```python
from build123d import *

# Parameters (mm, degrees)
F1_W     = 101.6
F1_H     = 101.6
F2_DEPTH = 50.8
F3_W     = 26.3578668237
F3_H     = 22.6122755557
F4_DEPTH = 50.8
F5_R     = 17.6293811016
F6_DEPTH = 50.8
F8_DEPTH = 50.8


# Not quite as in the source:
# - a variable given as a bare number and used for a length is read in inches; the dataset says mm whatever the document's units were


with BuildPart() as f2:
    # F1 (on Front) → F2 (new body, symmetric)
    with BuildSketch(Plane.XZ):
        Rectangle(F1_W, F1_H)
    extrude(amount=F2_DEPTH, both=True)

    # F3 (on face) → F4 (cut)
    with BuildSketch(Plane.XY.offset(50.8)):
        Rectangle(F3_W, F3_H)
    extrude(amount=-F4_DEPTH, mode=Mode.SUBTRACT)

    # F5 (on face) → F6 (cut)
    with BuildSketch(Plane(origin=(0, 0, -50.8), x_dir=(1, 0, 0), z_dir=(0, 0, -1))):
        with Locations((0, 1.7344856169)):
            Circle(F5_R)
    extrude(amount=-F6_DEPTH, mode=Mode.SUBTRACT)

    # F7 (on face) → F8 (cut)
    with BuildSketch(Plane(origin=(-50.8, 0, 0), x_dir=(0, -1, 0), z_dir=(-1, 0, 0))):
        Polygon((26.357864961, -15.2177204305), (26.357864961, 15.2177204305), (0, 30.435440861), (-26.357864961, 15.2177204305), (-26.357864961, -15.2177204305), (0, -30.435440861), align=None)
    extrude(amount=-F8_DEPTH, mode=Mode.SUBTRACT)


solid = f2.part
```
CAD build for the part. Positions are in the model's coordinates, mm. A direction names the side the tool comes from. Coordinates: 2 decimals unless noted, no trailing zeros. Write each loop counter-clockwise with the first axis right and the second up, starting at its lowest first coordinate (ties: lowest second). Pieces come first, ordered by that corner, then holes. Notation, with made-up numbers: (58, 74.25) -> (68, 74.25) arc R20 cw to (68, 87.25) -> close; hole circle Ø1 at (52, 20.5). An arc over 180 degrees is marked (long way). Use CSV: the item, a comma, the result in double quotes. Start each with the question number.
Item 1: Band-saw the part on B-B, the plane y = -6. Write the cut outline in (x, z), plus the area to 3 significant figures.
Item 2: Drop flat-ended pins along their axis: P1, Ø1.4, axis at x = 7.5, y = 13, coming from the -Z side; P2, Ø18, axis at y = -4, z = 15.5, coming from the -X side. Give the stop position or say it passes through.
Item 3: Band-saw the part on C-C, the plane x = -44. Write the cut outline in (y, z), plus the area to 3 significant figures.
Item 4: Band-saw the part on D-D, the plane z = 18. Write the cut outline in (x, y), plus the area to 3 significant figures.
Item 5: Band-saw the part on A-A, the plane z = 1.5. Write the cut outline in (x, y).
Item 6: Tool access for faces 4 (the flat face through (3, -11.306, 31)), 5 (the flat face through (-31.4, -12.994, -22.933)), 6 (the flat face through (-50.8, 22, 22)): list every direction of +Z, -Z, +X, -X, +Y, -Y with a clear straight run to the whole face (end or side of a thin tool).
Item 7: Wall check: probe 1 along X at (y, z) = (0.5, 40); probe 2 along Y at (x, z) = (0, -26.5); probe 3 along Y at (x, z) = (-7.5, 9). Give the ranges that are in metal, low to high.
Item 8: Two-plate mould, pull along Z, no slides. Class faces 1 (the flat face through (5, 13, 0)), 2 (the flat face through (-1, -50.8, 1)), 3 (the flat face through (0, -19, 3)): +Z half, -Z half, draft (parallel to the pull), parting line (faces both ways), or undercut.
Response values:
1,outline,"(-50.8, -50.8) -> (-17.11, -50.8) -> (-17.11, -26.97) -> (-50.8, -26.97) -> close; (-50.8, 26.97) -> (-13.18, 26.97) -> (-13.18, 50.8) -> (-50.8, 50.8) -> close; (13.18, 0) -> (17.11, 0) -> (17.11, -50.8) -> (50.8, -50.8) -> (50.8, 50.8) -> (13.18, 50.8) -> close"
1,area,"5,320 mm2"
2,P1,"stops at z = 0"
2,P2,"stops at x = 0"
3,outline,"(-50.8, -50.8) -> (50.8, -50.8) -> (50.8, 50.8) -> (-50.8, 50.8) -> close; hole (-26.36, -15.22) -> (0, -30.44) -> (26.36, -15.22) -> (26.36, 15.22) -> (0, 30.44) -> (-26.36, 15.22) -> close"
3,area,"7,920 mm2"
4,outline,"(-50.8, -50.8) -> (50.8, -50.8) -> (50.8, 50.8) -> (-50.8, 50.8) -> (-50.8, 21.54) -> (0, 21.54) -> (0, 11.31) -> (13.18, 11.31) -> (13.18, -11.31) -> (0, -11.31) -> (0, -21.54) -> (-50.8, -21.54) -> close"
4,area,"7,840 mm2"
5,outline,"(-50.8, -50.8) -> (50.8, -50.8) -> (50.8, 50.8) -> (-50.8, 50.8) -> (-50.8, 26.36) -> (0, 26.36) -> (0, 11.31) -> (13.18, 11.31) -> (13.18, -11.31) -> (0, -11.31) -> (0, -26.36) -> (-50.8, -26.36) -> close"
6,face 4,"+Z, -Z"
6,face 5,"-X"
6,face 6,"+Z, -Z, -X, +Y, -Y"
7,probe 1,"x = -50.8 to -13.18, 13.18 to 50.8"
7,probe 2,"y = -50.8 to -19.36, 15.89 to 50.8"
7,probe 3,"y = -50.8 to -26.36, 26.36 to 50.8"
8,face 1,"-Z half"
8,face 2,"draft"
8,face 3,"undercut"
